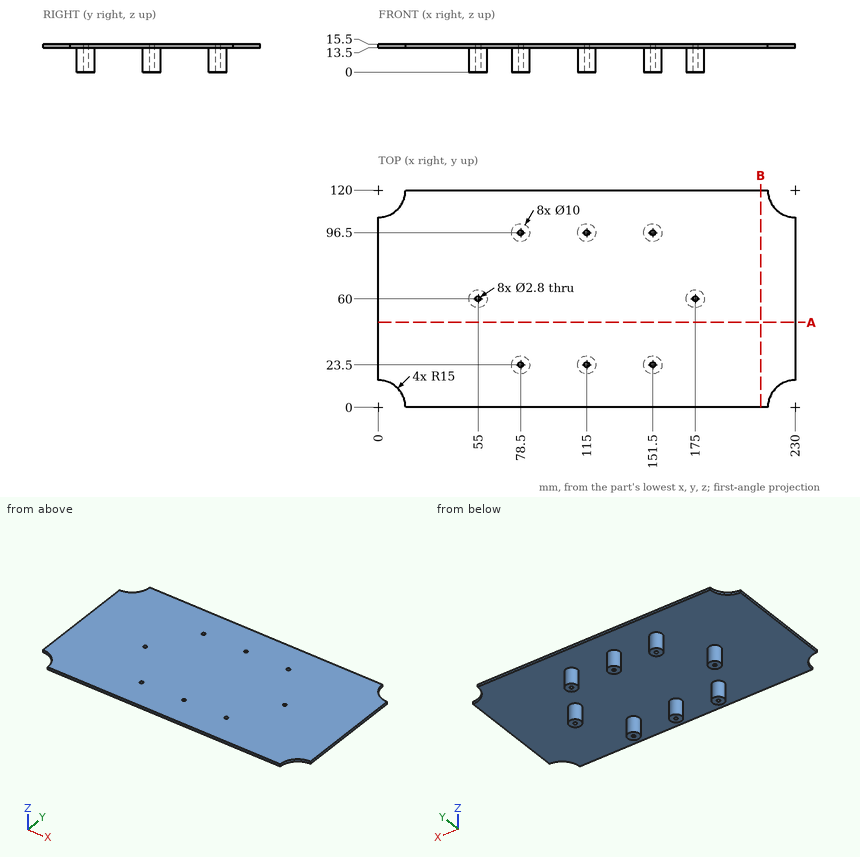
Design review of the part shown in the three views and the two pictorial views. Dimensions are in mm from the part's minimum x, y and z. Give positions to 0.01 mm unless a question says otherwise; leave off trailing zeros. Write each loop counter-clockwise with the first axis right and the second up, starting at its lowest first coordinate (ties: lowest second). Pieces come first, ordered by that corner, then holes. Notation, with made-up numbers: (17, 14.25) - (66, 14.25) arc R30 cw to (66, 41.25) - close; hole circle Ø3 at (27, 12). An arc over 180 degrees is marked (long way). Return JSON: item names as keys, results as strings. Group by question number.
(1) We need section B-B, the plane x = 211. Give the boundary of the cut face in (y, z), then the cut area to 3 significant figures.
(2) To check wall thickness, follow probe 1 along Y at (x, z) = (78.5, 5.5); probe 2 along Y at (x, z) = (175, 5.75); probe 3 along Z at (x, y) = (179.5, 91.5). State the ranges of each line that lie inside material, in increasing order.
(3) Insertion check: pin 1 (5 mm diameter, centred on x = 147, z = 9, fed in from +Y); pin 2 (1.5 mm diameter, centred on x = 150.5, z = 2, fed in from -Y); pin 3 (2 mm diameter, centred on x = 78.5, y = 96.5, fed in from -Z); pin 4 (8 mm diameter, centred on x = 30, y = 92.5, fed in from -Z). Each pin has a flat end and moves straight along its axis. Give the tip position at first contact, or say it passes through.
(4) We need section A-A, the plane y = 47. Give the boundary of the cut face in (x, z).
Reported:
{
 "1": {"outline": "(0, 13.5) - (120, 13.5) - (120, 15.5) - (0, 15.5) - close", "area": "240 mm2"},
 "2": {"probe 1": "y = 18.5 to 22.1, 24.9 to 28.5, 91.5 to 95.1, 97.9 to 101.5", "probe 2": "y = 55 to 58.6, 61.4 to 65", "probe 3": "z = 13.5 to 15.5"},
 "3": {"pin 1": "stops at y = 101.08", "pin 2": "stops at y = 18.51", "pin 3": "passes through", "pin 4": "stops at z = 13.5"},
 "4": {"outline": "(0, 13.5) - (230, 13.5) - (230, 15.5) - (0, 15.5) - close"}
}
